Could you check a few things on this model? Use its own coordinates, in mm. A direction names the side the tool comes from. Coordinates: 2 decimals unless noted, no trailing zeros. Loops run counter-clockwise (first coordinate to the right, second up) from the corner with the lowest first, then second, coordinate; pieces in that order, holes last.
1) For faces 1 (the face through (-1, 3.175, 10)), 2 (the face through (13.652, 0, 15)), which set-ups out of +Z, -Z, +X, -X, +Y, -Y let a thin tool reach every point of the face, with its end or its side?
2) Thinking about a two-plate mould opening in X: for faces 3 (the face through (3, 0, 25.4)), 4 (the face through (-21.908, 0, 15)), 5 (the face through (-63.5, 0, 12)), which applies, released by +X, released by -X, zero draft, split by the parting line, or undercut?
3) Imagine slicing it at B-B on x = -7.5. Please give me the cut outline in (y, z) (3 decimals), plus the area to 3 significant figures.
4) Imagine slicing it at A-A on z = 19. Give the number of separate pieces and of enclosed holes in the cut face, plus the area to 3 significant figures.
5) If I drill on line 1 along X through (y, z) = (2.5, 9.5); line 2 along X through (y, z) = (0.75, 15.75); line 3 along Y through (x, z) = (-57.25, 3.81) (3 decimals), over which ranges is the centre line in solid material (lowest first)?
6) Will these pins go through, and if not, where does the flat tip stop? P1, Ø1.9, axis at x = -19.5, y = 0, coming from the +Z side; P2, Ø2.5, axis at y = 0, z = 3.81, coming from the -X side.
```python
from build123d import *

# Parameters (mm, degrees)
F0_W           = 127
F0_H           = 6.35
F1_DEPTH       = 25.4
F2_W           = 3.81
F2_H           = 19.05
F2_W_2         = 8.5344
F2_H_2         = 7.874
F3_DEPTH       = 6.35
F4_R           = 1.905
F7_D           = 2.7051
F7_DEPTH       = 14.224
F7_TIP         = 0.8126940303
F7_ON_F6_D     = 2.7051
F7_ON_F6_DEPTH = 14.224
F7_ON_F6_TIP   = 0.8126940303
F8_D           = 2.7051
F8_DEPTH       = 8.89
F8_TIP         = 0.8126940303


with BuildPart() as f1:
    # F0 (on Top) → F1 (new body)
    with BuildSketch(Plane.XY):
        Rectangle(F0_W, F0_H)
    extrude(amount=F1_DEPTH)

    # F2 (on face) → F3 (cut, through all)
    with BuildSketch(Plane.XZ.offset(3.175)):
        with Locations((-51.7525, 15.875)):
            Rectangle(F2_W, F2_H)
        with Locations((-20.0025, 15.875)):
            Rectangle(F2_W, F2_H)
        with Locations((11.7475, 15.875)):
            Rectangle(F2_W, F2_H)
        with Locations((43.4975, 15.875)):
            Rectangle(F2_W, F2_H)
        with Locations((-39.0652, 21.463)):
            Rectangle(F2_W_2, F2_H_2)
        with Locations((-7.8232, 21.463)):
            Rectangle(F2_W_2, F2_H_2)
        with Locations((23.4188, 21.463)):
            Rectangle(F2_W_2, F2_H_2)
        with Locations((54.6608, 21.463)):
            Rectangle(F2_W_2, F2_H_2)
    extrude(amount=-F3_DEPTH, mode=Mode.SUBTRACT)

    # F4
    f4_edges = [f1.edges().sort_by_distance(p)[0] for p in [
        (-53.6575, 0, 25.4),
        (-49.8475, 0, 25.4),
        (-21.9075, 0, 25.4),
        (-18.0975, 0, 25.4),
        (9.8425, 0, 25.4),
        (13.6525, 0, 25.4),
        (41.5925, 0, 25.4),
        (45.4025, 0, 25.4),
        (-43.3324, 0, 25.4),
        (-34.798, 0, 25.4),
        (-12.0904, 0, 25.4),
        (-3.556, 0, 25.4),
        (19.1516, 0, 25.4),
        (27.686, 0, 25.4),
        (50.3936, 0, 25.4),
        (58.928, 0, 25.4),
        (63.5, 0, 25.4),
        (-63.5, 0, 25.4),
    ]]
    fillet(f4_edges, radius=F4_R)

    # F7
    with Locations(Plane(origin=(0, 0, 0), x_dir=(1, 0, 0), z_dir=(0, 0, -1))):
        with Locations((-38.1, 0), (38.1, 0)):
            Hole(F7_D / 2, depth=F7_DEPTH)
            with Locations((0, 0, -(F7_DEPTH + F7_TIP / 2))):  # 118° drill point
                Cone(0, F7_D / 2, F7_TIP, mode=Mode.SUBTRACT)

    # F7 on F6
    with Locations(Plane(origin=(-63.5, 0, 0), x_dir=(0, -1, 0), z_dir=(-1, 0, 0))):
        with Locations((0, 3.81)):
            Hole(F7_ON_F6_D / 2, depth=F7_ON_F6_DEPTH)
            with Locations((0, 0, -(F7_ON_F6_DEPTH + F7_ON_F6_TIP / 2))):  # 118° drill point
                Cone(0, F7_ON_F6_D / 2, F7_ON_F6_TIP, mode=Mode.SUBTRACT)

    # F8
    with Locations(Plane(origin=(-63.5, 0, 0), x_dir=(0, -1, 0), z_dir=(-1, 0, 0))):
        with Locations((0, 16.51)):
            Hole(F8_D / 2, depth=F8_DEPTH)
            with Locations((0, 0, -(F8_DEPTH + F8_TIP / 2))):  # 118° drill point
                Cone(0, F8_D / 2, F8_TIP, mode=Mode.SUBTRACT)


solid = f1.part
```
Filled in:
1. face 1: +Z, -Z, +X, -X, +Y
1. face 2: +Z, +Y, -Y
2. face 3: zero draft
2. face 4: undercut
2. face 5: released by -X
3. outline: (-3.175, 0) - (3.175, 0) - (3.175, 17.526) - (-3.175, 17.526) - close
3. area: 111 mm2
4. separate pieces: 9
4. enclosed holes: 0
4. area: 493 mm2
5. line 1: x = -63.5 to -53.66, -49.85 to -21.91, -18.1 to 9.84, 13.65 to 41.59, 45.4 to 63.5
5. line 2: x = -54.44 to -53.66, -49.85 to -21.91, -18.1 to 9.84, 13.65 to 41.59, 45.4 to 63.5
5. line 3: y = -3.175 to -1.353, 1.353 to 3.175
6. P1: stops at z = 6.35
6. P2: stops at x = -49.21
